from build123d import *

# Parameters (mm, degrees)
BOSS_EXTRUDE1_DEPTH = 50.8
CUT_EXTRUDE1_DEPTH  = 2.27


with BuildPart() as part:
    # Sketch2 → Boss-Extrude1 (new body, symmetric)
    with BuildSketch(Plane(origin=(0, 0, 0), x_dir=(1, 0, 0), z_dir=(0, 1, 0))):
        with BuildLine():
            Line((-5.969, 0), (19.431, 0))
            ThreePointArc((19.431, 0), (19.700407684, -0.111592316), (19.812, -0.381))
            Line((19.812, -0.381), (19.812, -0.889))
            ThreePointArc((19.812, -0.889), (19.700407684, -1.158407684), (19.431, -1.27))
            Line((19.431, -1.27), (1.016, -1.27))
            ThreePointArc((1.016, -1.27), (0.746592316, -1.381592316), (0.635, -1.651))
            Line((0.635, -1.651), (0.635, -12.827))
            ThreePointArc((0.635, -12.827), (0.746592316, -13.096407684), (1.016, -13.208))
            Line((1.016, -13.208), (1.40496875, -13.208))
            ThreePointArc((1.40496875, -13.208), (1.539672592, -13.183392866), (1.656976563, -13.11275))
            ThreePointArc((1.656976563, -13.11275), (3.556, -13.97), (1.656976563, -14.82725))
            ThreePointArc((1.656976563, -14.82725), (1.539672592, -14.756607134), (1.40496875, -14.732))
            Line((1.40496875, -14.732), (-1.40496875, -14.732))
            ThreePointArc((-1.40496875, -14.732), (-1.539672592, -14.756607134), (-1.656976563, -14.82725))
            ThreePointArc((-1.656976563, -14.82725), (-3.556, -13.97), (-1.656976563, -13.11275))
            ThreePointArc((-1.656976563, -13.11275), (-1.539672592, -13.183392866), (-1.40496875, -13.208))
            Line((-1.40496875, -13.208), (-1.016, -13.208))
            ThreePointArc((-1.016, -13.208), (-0.746592316, -13.096407684), (-0.635, -12.827))
            Line((-0.635, -12.827), (-0.635, -1.651))
            ThreePointArc((-0.635, -1.651), (-0.746592316, -1.381592316), (-1.016, -1.27))
            Line((-1.016, -1.27), (-5.969, -1.27))
            ThreePointArc((-5.969, -1.27), (-6.238407684, -1.158407684), (-6.35, -0.889))
            Line((-6.35, -0.889), (-6.35, -0.381))
            ThreePointArc((-6.35, -0.381), (-6.238407684, -0.111592316), (-5.969, 0))
        make_face()
    extrude(amount=BOSS_EXTRUDE1_DEPTH, both=True)

    # Sketch3 → Cut-Extrude1 (cut, through all)
    with BuildSketch(Plane.XY.offset(1.27)):
        with BuildLine():
            Line((11.08075, 2.38125), (12.66825, 2.38125))
            ThreePointArc((12.66825, 2.38125), (15.0495, 0), (12.66825, -2.38125))
            Line((12.66825, -2.38125), (11.08075, -2.38125))
            ThreePointArc((11.08075, -2.38125), (8.6995, 0), (11.08075, 2.38125))
        make_face()
    extrude(amount=-CUT_EXTRUDE1_DEPTH, mode=Mode.SUBTRACT)


solid = part.part
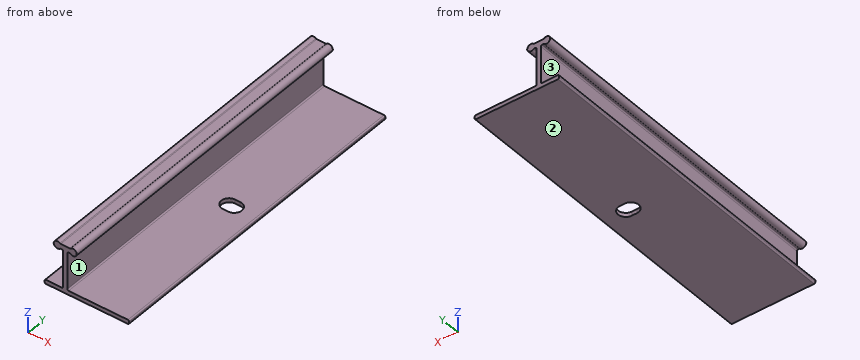
Geometry: final body of the model. Coordinates: model frame, mm. Face numbers are marked on the shaded views. Give positions to 0.01 mm unless a question says otherwise; leave off trailing zeros. Loops run counter-clockwise (first coordinate to the right, second up) from the corner with the lowest first, then second, coordinate; pieces in that order, holes last. Notation, with made-up numbers: M 75.5,12 L 81.5,12 A16 ccw 81.5,31 Z; hole C -34.75,29.25 d10. An arc over 180 degrees is marked long. Put each result on its own line as item: value. Start each with the question number.
1) Contact query for flat-ended pins moving along their axis: pin 1 (10 mm diameter, centred on x = 3.5, y = -3.5, fed in from -Z); pin 2 (3.5 mm diameter, centred on y = 11, z = 9, fed in from +X) (3 decimals); pin 3 (8 mm diameter, centred on x = 10, z = 7.5, fed in from -Y); pin 4 (9 mm diameter, centred on x = 11.5, y = -2.5, fed in from +Z). Output: stop coordinate, or through.
2) Ray query, line 1 along Z through (x, y) = (-2.5, 20); line 2 along X through (y, z) = (23, 10.75) (3 decimals); line 3 along Z through (x, y) = (4.25, 18.5). Return the intervals inside material, ascending.
3) Cut plane B-B (x = 16.75). Output: boundary loops of the cut face in (y, z), then the cut area to 3 significant figures.
4) Pull-direction query (Z, two-part tool) for the marked faces 1, 2 and 3; classes: pulls with the +Z half, pulls with the -Z half, needs draft (parallel to the pull), parting line crosses it, or undercut.
Verdict:
1. pin 1: z = 0
1. pin 2: x = 0.635
1. pin 3: through
1. pin 4: z = 1.27
2. line 1: 0 to 1.27, 12.83 to 15.11
2. line 2: -0.635 to 0.635
2. line 3: 0 to 1.27
3. outline: M -50.8,0 L 50.8,0 L 50.8,1.27 L -50.8,1.27 Z
3. area: 129 mm2
4. face 1: undercut
4. face 2: pulls with the -Z half
4. face 3: undercut
